Here's how the part is built. I have some questions about the finished solid (model axes, mm). Face numbers are marked on the shaded views. A direction names the side the tool comes from. Coordinates: 2 decimals unless noted, no trailing zeros. Write each loop counter-clockwise with the first axis right and the second up, starting at its lowest first coordinate (ties: lowest second). Pieces come first, ordered by that corner, then holes. Notation, with made-up numbers: M 33.5,53 L 89.5,53 A18 ccw 89.5,73 Z; hole C -14.5,-37 d6. An arc over 180 degrees is marked long. Use one line per item in the form item = value. Start each with the question number.
1. I'm going to push a flat-ended pin straight in: pin 1 Ø4 at (x, y) = (-83, 7) entering from -Z. Where does the tip first touch, or does it pass through?
2. I want a section at B-B, the plane x = -109. List the corners of the cut face in (y, z) for me, plus the area to 3 significant figures.
3. I want a section at A-A, the plane x = -96. List the corners of the cut face in (y, z) for me.
4. Thinking about a two-plate mould opening in Y: for the marked faces 3, 4, 5 and 6, which applies, released by +Y, released by -Y, zero draft, split by the parting line, or undercut?
5. Please list where these lines run through material, in increasing order: line 1 along Y through (x, z) = (-109, 53.55); line 2 along Y through (x, z) = (-85.5, 51.2); line 3 along X through (y, z) = (24, 51.5). Write a range as [from, to].
6. I want a section at C-C, the plane y = 18. List the corners of the cut face in (x, z) for me.
7. On a 3-axis mill with a long thin cutter (end or side, diameter ignored), from which of +Z, -Z, +X, -X, +Y, -Y can I reach the whole of each face in a straight line? I mean the marked faces 1 and 2. Say none if no direction works.
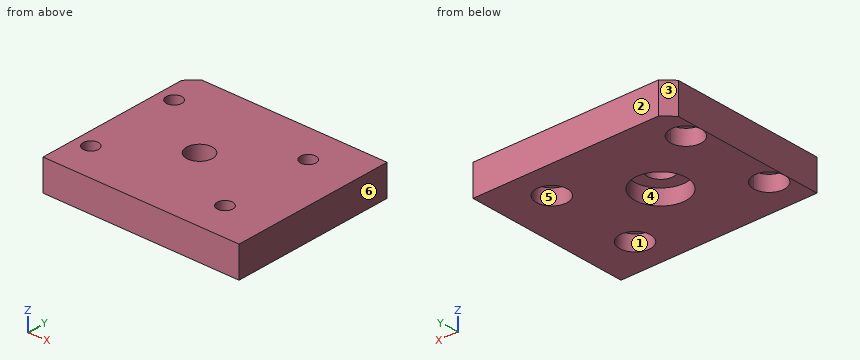
from build123d import *

# Parameters (mm, degrees)
CYLINDER882_R     = 5
CYLINDER882_DEPTH = 3
CYLINDER891_R     = 2.5
CYLINDER891_DEPTH = 20
CYLINDER883_R     = 1.5
CYLINDER883_DEPTH = 20
CYLINDER885_R     = 1.5
CYLINDER885_DEPTH = 20
CYLINDER886_R     = 1.5
CYLINDER886_DEPTH = 20
CYLINDER884_R     = 1.5
CYLINDER884_DEPTH = 20
CYLINDER887_R     = 3
CYLINDER887_DEPTH = 3
CYLINDER888_R     = 3
CYLINDER888_DEPTH = 3
CYLINDER890_R     = 3
CYLINDER890_DEPTH = 3
CYLINDER889_R     = 3
CYLINDER889_DEPTH = 3
BOX422_W          = 38
BOX422_H          = 32
BOX422_DEPTH      = 6
CHAMFER001_SIZE   = 2


with BuildPart() as obj1:
    # Cylinder882 → Cylinder882 (new body)
    with BuildSketch(Plane(origin=(-96, 16, 50), x_dir=(1, 0, 0), z_dir=(0, 0, 1))):
        Circle(CYLINDER882_R)
    extrude(amount=CYLINDER882_DEPTH)


with BuildPart() as obj2:
    # Cylinder891 → Cylinder891 (new body)
    with BuildSketch(Plane(origin=(-96, 16, 50), x_dir=(1, 0, 0), z_dir=(0, 0, 1))):
        Circle(CYLINDER891_R)
    extrude(amount=CYLINDER891_DEPTH)


with BuildPart() as obj3:
    # Cylinder883 → Cylinder883 (new body)
    with BuildSketch(Plane(origin=(-83, 25, 54), x_dir=(1, 0, 0), z_dir=(0, 0, 1))):
        Circle(CYLINDER883_R)
    extrude(amount=CYLINDER883_DEPTH)


with BuildPart() as obj4:
    # Cylinder885 → Cylinder885 (new body)
    with BuildSketch(Plane(origin=(-109, 7, 54), x_dir=(1, 0, 0), z_dir=(0, 0, 1))):
        Circle(CYLINDER885_R)
    extrude(amount=CYLINDER885_DEPTH)


with BuildPart() as obj5:
    # Cylinder886 → Cylinder886 (new body)
    with BuildSketch(Plane(origin=(-109, 25, 54), x_dir=(1, 0, 0), z_dir=(0, 0, 1))):
        Circle(CYLINDER886_R)
    extrude(amount=CYLINDER886_DEPTH)


with BuildPart() as compound491:
    # Cylinder884 → Cylinder884 (new body)
    with BuildSketch(Plane(origin=(-83, 7, 54), x_dir=(1, 0, 0), z_dir=(0, 0, 1))):
        Circle(CYLINDER884_R)
    extrude(amount=CYLINDER884_DEPTH)

    # Compound491: union obj3, obj4, obj5
    add(obj3.part)
    add(obj4.part)
    add(obj5.part)


with BuildPart() as compound491_1:
    # Compound491 placement: moved
    add(compound491.part.moved(Location((0, 0, -4))))


with BuildPart() as obj6:
    # Cylinder887 → Cylinder887 (new body)
    with BuildSketch(Plane(origin=(-83, 25, 54), x_dir=(1, 0, 0), z_dir=(0, 0, 1))):
        Circle(CYLINDER887_R)
    extrude(amount=CYLINDER887_DEPTH)


with BuildPart() as obj7:
    # Cylinder888 → Cylinder888 (new body)
    with BuildSketch(Plane(origin=(-109, 7, 54), x_dir=(1, 0, 0), z_dir=(0, 0, 1))):
        Circle(CYLINDER888_R)
    extrude(amount=CYLINDER888_DEPTH)


with BuildPart() as obj8:
    # Cylinder890 → Cylinder890 (new body)
    with BuildSketch(Plane(origin=(-109, 25, 54), x_dir=(1, 0, 0), z_dir=(0, 0, 1))):
        Circle(CYLINDER890_R)
    extrude(amount=CYLINDER890_DEPTH)


with BuildPart() as compound492:
    # Cylinder889 → Cylinder889 (new body)
    with BuildSketch(Plane(origin=(-83, 7, 54), x_dir=(1, 0, 0), z_dir=(0, 0, 1))):
        Circle(CYLINDER889_R)
    extrude(amount=CYLINDER889_DEPTH)

    # Compound492: union obj6, obj7, obj8
    add(obj6.part)
    add(obj7.part)
    add(obj8.part)


with BuildPart() as compound492_1:
    # Compound492 placement: moved
    add(compound492.part.moved(Location((0, 0, -4))))


with BuildPart() as obj9:
    # Box422 → Box422 (new body)
    with BuildSketch(Plane(origin=(-112, 0, 50), x_dir=(1, 0, 0), z_dir=(0, 0, 1))):
        with Locations((19, 16)):
            Rectangle(BOX422_W, BOX422_H)
    extrude(amount=BOX422_DEPTH)

    # Cut394: cut Compound492
    add(compound492_1.part, mode=Mode.SUBTRACT)

    # Cut395: cut Compound491
    add(compound491_1.part, mode=Mode.SUBTRACT)

    # Cut396: cut obj2
    add(obj2.part, mode=Mode.SUBTRACT)

    # Cut397: cut obj1
    add(obj1.part, mode=Mode.SUBTRACT)

    # Chamfer001
    chamfer001_edges = [obj9.edges().sort_by_distance(p)[0] for p in [
        (-112, 32, 53),
    ]]
    chamfer(chamfer001_edges, length=CHAMFER001_SIZE)


solid = obj9.part
Answer list:
q1.pin_1 = 53
q2.outline = M 0,50 L 4,50 L 4,53 L 5.5,53 L 5.5,56 L 0,56 Z; M 8.5,53 L 10,53 L 10,50 L 22,50 L 22,53 L 23.5,53 L 23.5,56 L 8.5,56 Z; M 26.5,53 L 28,53 L 28,50 L 32,50 L 32,56 L 26.5,56 Z
q2.area = 138 mm²
q3.outline = M 0,50 L 11,50 L 11,53 L 13.5,53 L 13.5,56 L 0,56 Z; M 18.5,53 L 21,53 L 21,50 L 32,50 L 32,56 L 18.5,56 Z
q4.face_3 = released by +Y
q4.face_4 = undercut
q4.face_5 = undercut
q4.face_6 = zero draft
q5.line_1 = [0, 5.5], [8.5, 23.5], [26.5, 32]
q5.line_2 = [0, 5.34], [8.66, 23.34], [26.66, 32]
q5.line_3 = [-112, -111.83], [-106.17, -85.83], [-80.17, -74]
q6.outline = M -112,50 L -100.58,50 L -100.58,53 L -97.5,53 L -97.5,56 L -112,56 Z; M -94.5,53 L -91.42,53 L -91.42,50 L -74,50 L -74,56 L -94.5,56 Z
q7.face_1 = -Z
q7.face_2 = +Z, -Z, +X, -X, +Y
